Geometry check sheet. Reference: drawing and pictorial views, mm from the part's lowest x, y, z. Round coordinates to 2 decimals unless told otherwise and drop trailing zeros. Order: outer loops, then holes, each group sorted by start corner. A loop starts at its lowest first (then second) coordinate and runs counter-clockwise, first axis right, second up.
(1) Thickness scan on L1, parallel to Y at x = 88.9, z = 1.55; L2, parallel to X at y = 21, z = 3.1; L3, parallel to X at y = 19.5, z = 2.95. Record the ranges inside material, lowest first.
(2) Cross-section at B-B on y = 29. Enter the section's corners in (x, z).
(3) Cross-section at A-A on x = 88.9. Enter the section's corners in (y, z).
(4) Cross-section at C-C on z = 1.2. Enter the section's corners in (x, y), and give its area (3 significant figures).
(5) Gauge pin test, flat end, axial feed: P1, Ø5, axis at x = 140, y = 12.5, coming from the -Z side. Record the tip position at first contact, or that the pin passes through.
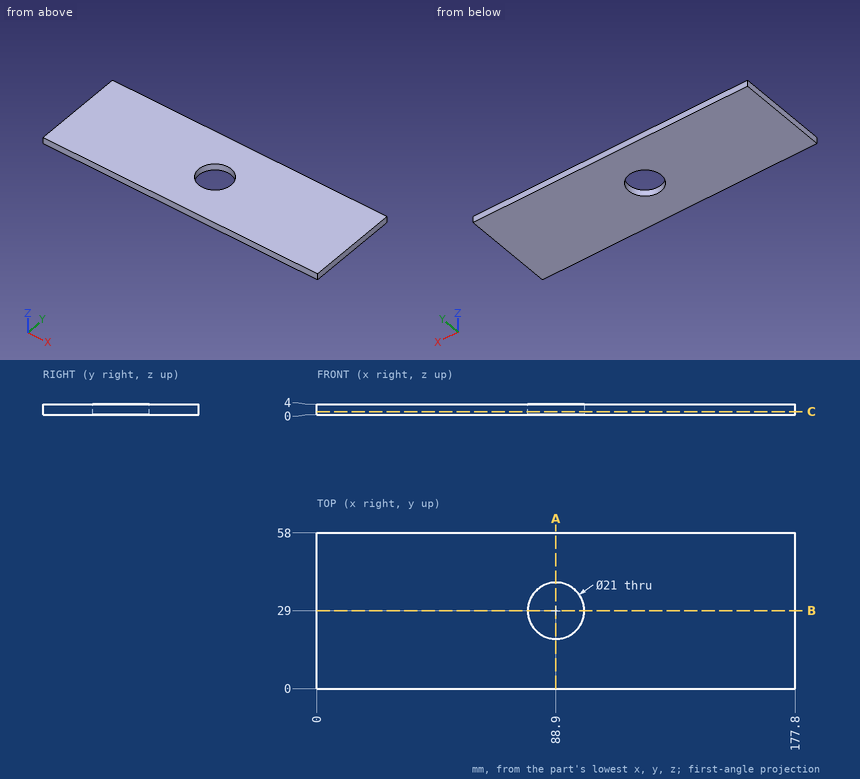
Found:
1. L1: y = 0 to 18.5, 39.5 to 58
1. L2: x = 0 to 82.1, 95.7 to 177.8
1. L3: x = 0 to 84.43, 93.37 to 177.8
2. outline: (0, 0) - (78.4, 0) - (78.4, 4) - (0, 4) - close; (99.4, 0) - (177.8, 0) - (177.8, 4) - (99.4, 4) - close
3. outline: (0, 0) - (18.5, 0) - (18.5, 4) - (0, 4) - close; (39.5, 0) - (58, 0) - (58, 4) - (39.5, 4) - close
4. outline: (0, 0) - (177.8, 0) - (177.8, 58) - (0, 58) - close; hole circle Ø21 at (88.9, 29)
4. area: 9,970 mm2
5. P1: stops at z = 0
